The model under review builds one solid part; all positions refer to its coordinate system, in mm. Face numbers are marked on the shaded views. Round coordinates to 2 decimals unless told otherwise and drop trailing zeros. Loops run counter-clockwise (first coordinate to the right, second up) from the corner with the lowest first, then second, coordinate; pieces in that order, holes last. Notation, with made-up numbers: M 15,83 L 24,83 A27 cw 24,106 Z; hole C 87,75 d2. An arc over 180 degrees is marked long. Use a Markdown table: item, result. Add a question column.
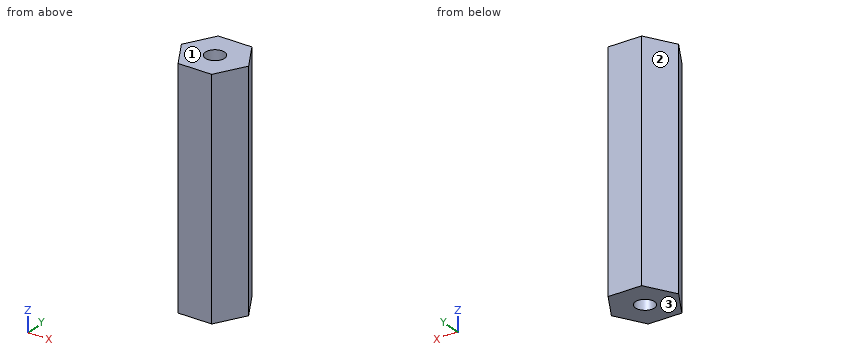
```python
from build123d import *

# Parameters (mm, degrees)
BOSS_EXTRU_1_DEPTH      = 40
ESQUISSE2_R             = 1.65
ENL_V_MAT_EXTRU_1_DEPTH = 9
ENL_V_START             = -31
ESQUISSE2_2_R           = 1.65
ENL_V_MAT_EXTRU_2_DEPTH = 9


with BuildPart() as part:
    # Esquisse1 → Boss.-Extru.1 (new body)
    with BuildSketch(Plane.XY):
        Polygon((5.773502692, 0), (2.886751346, 5), (-2.886751346, 5), (-5.773502692, 0), (-2.886751346, -5), (2.886751346, -5), align=None)
    extrude(amount=BOSS_EXTRU_1_DEPTH)

    # Esquisse2 → Enlèv. mat.-Extru.1 (cut)
    with BuildSketch(Plane.XY.offset(40)):
        Circle(ESQUISSE2_R)
    extrude(amount=-ENL_V_MAT_EXTRU_1_DEPTH, mode=Mode.SUBTRACT)

    # Esquisse2<2> → Enlèv. mat.-Extru.2 (cut)
    with BuildSketch(Plane.XY.offset(40).offset(ENL_V_START)):
        Circle(ESQUISSE2_2_R)
    extrude(amount=-ENL_V_MAT_EXTRU_2_DEPTH, mode=Mode.SUBTRACT)


solid = part.part
```
(1) To check wall thickness, follow probe 1 along Y at (x, z) = (0, 6); probe 2 along Z at (x, y) = (-0.25, -0.75); probe 3 along X at (y, z) = (0.25, 36). State the ranges of each line that lie inside material, in increasing order.
(2) Insertion check: pin 1 Ø2.5 at (x, y) = (0, 0) entering from +Z; pin 2 Ø3 at (y, z) = (3.5, 11) entering from -X. Each pin has a flat end and moves straight along its axis. Give the tip position at first contact, or say it passes through.
(3) Consider section C-C, the plane y = 1.25. Give the boundary of the cut face in (x, z), then the cut area to 3 significant figures.
(4) Draft analysis for pull direction Z (two halves, no side actions). For the marked faces 1, 2 and 3, state which applies: released by +Z, released by -Z, zero draft, split by the parting line, or undercut.
(5) Consider section D-D, the plane z = 14.5. Give the boundary of the cut face in (x, y), then the cut area to 3 significant figures.
(6) Consider section B-B, the plane x = 0. Give the boundary of the cut face in (y, z).
(7) Consider section A-A, the plane z = 5.5. Give the boundary of the cut face in (x, y).
Found:
| question | item | result |
|---|---|---|
| 1 | probe 1 | y = -5 to -1.65, 1.65 to 5 |
| 1 | probe 2 | z = 9 to 31 |
| 1 | probe 3 | x = -5.63 to -1.63, 1.63 to 5.63 |
| 2 | pin 1 | stops at z = 31 |
| 2 | pin 2 | stops at x = -4.62 |
| 3 | outline | M -5.05,0 L -1.08,0 L -1.08,9 L 1.08,9 L 1.08,0 L 5.05,0 L 5.05,40 L 1.08,40 L 1.08,31 L -1.08,31 L -1.08,40 L -5.05,40 Z |
| 3 | area | 365 mm^2 |
| 4 | face 1 | released by +Z |
| 4 | face 2 | zero draft |
| 4 | face 3 | released by -Z |
| 5 | outline | M -5.77,0 L -2.89,-5 L 2.89,-5 L 5.77,0 L 2.89,5 L -2.89,5 Z |
| 5 | area | 86.6 mm^2 |
| 6 | outline | M -5,0 L -1.65,0 L -1.65,9 L 1.65,9 L 1.65,0 L 5,0 L 5,40 L 1.65,40 L 1.65,31 L -1.65,31 L -1.65,40 L -5,40 Z |
| 7 | outline | M -5.77,0 L -2.89,-5 L 2.89,-5 L 5.77,0 L 2.89,5 L -2.89,5 Z; hole C 0,0 d3.3 |
